```python
from build123d import *

# Parameters (mm, degrees)
RESSALTO_EXTRUS_O1_DEPTH  = 5
RESSALTO_EXTRUS_O2_DEPTH  = 15.5
RESSALTO_EXTRUS_O3_DEPTH  = 15.5
RESSALTO_EXTRUS_O4_DEPTH  = 20
ESBO_O6_W                 = 5
ESBO_O6_H                 = 16.897720337
RESSALTO_EXTRUS_O5_DEPTH  = 23.2
ESBO_O7_W                 = 13.499987793
ESBO_O7_H                 = 16.897720337
RESSALTO_EXTRUS_O6_DEPTH  = 8
ESBO_O8_W                 = 2.000000014
ESBO_O8_H                 = 6.588073731
CORTE_EXTRUS_O1_DEPTH     = 93.188310305
CHANFRO2_SIZE             = 9
RESSALTO_EXTRUS_O8_DEPTH  = 4.5
RESSALTO_EXTRUS_O7_START  = -5.5
RESSALTO_EXTRUS_O7_DEPTH  = 6
CORTE_EXTRUS_O2_REACH     = 102.674
ESBO_O11_W                = 11.999984741
ESBO_O11_H                = 13.640792847
CORTE_EXTRUS_O4_REACH     = 108.65
ESBO_O13_R                = 1.6
RESSALTO_EXTRUS_O9_DEPTH  = 5
ESBO_O16_W                = 11.500915527
ESBO_O16_H                = 13.642723083
CORTE_EXTRUS_O5_DEPTH     = 101.673633611
RESSALTO_EXTRUS_O13_START = -15.5
ESBO_O18_W                = 32.102264404
ESBO_O18_H                = 11
RESSALTO_EXTRUS_O13_DEPTH = 77.5
ESBO_O27_W                = 32.102264404
ESBO_O27_H                = 11
CORTE_EXTRUS_O8_DEPTH     = 20.5
ESBO_O29_R                = 1.9
CORTE_EXTRUS_O9_DEPTH     = 2.5
ESBO_O30_R                = 1.9
CORTE_EXTRUS_O10_DEPTH    = 6
ESBO_O32_W                = 20
ESBO_O32_H                = 78
CORTE_EXTRUS_O11_DEPTH    = 88.462468019
ESBO_O33_R                = 1.75
CORTE_EXTRUS_O12_DEPTH    = 26
CORTE_EXTRUS_O13_START    = -6
CORTE_EXTRUS_O13_DEPTH    = 2.9
RESSALTO_EXTRUS_O20_DEPTH = 10
ESBO_O40_W                = 68.75
ESBO_O40_H                = 49.5
ESBO_O40_W_2              = 60.75
ESBO_O40_H_2              = 41.5
RESSALTO_EXTRUS_O21_DEPTH = 18.5
ESBO_O41_W                = 11.75
ESBO_O41_H                = 49.5
ESBO_O41_W_2              = 41.5
ESBO_O41_H_2              = 38.5
RESSALTO_EXTRUS_O22_DEPTH = 2
RESSALTO_EXTRUS_O23_DEPTH = 15.5
ESBO_O43_W                = 4
ESBO_O43_H                = 33.5
ESBO_O43_W_2              = 14
ESBO_O43_H_2              = 4
CORTE_EXTRUS_O14_DEPTH    = 18.5
RESSALTO_EXTRUS_O24_DEPTH = 20.5
ESBO_O45_R                = 1.8
CORTE_EXTRUS_O15_DEPTH    = 6
FILETE1_R                 = 4
FILETE2_R                 = 2


with BuildPart() as part:
    # Esboço2 → Ressalto-extrusão1 (new body)
    with BuildSketch(Plane.XY):
        Polygon((0, 0), (0, -60.9), (-20, -60.9), (-20, -25.9), (-15.5, -15.9), (-15.5, 0), align=None)
    extrude(amount=RESSALTO_EXTRUS_O1_DEPTH)

    # Esboço3 → Ressalto-extrusão2 (add)
    with BuildSketch(Plane(origin=(0, 0, 0), x_dir=(0, 0, -1), z_dir=(1, 0, 0))):
        with BuildLine():
            ThreePointArc((6.102294922, 14.1), (-2.871049482, 9.744626932), (-5, 0))
            Line((-5, 0), (0, 0))
            ThreePointArc((0, 0), (1.788130128, 4.313492501), (6.102294922, 6.1))
            Line((6.102294922, 6.1), (30.102294922, 6.1))
            ThreePointArc((30.102294922, 6.099999986), (40.781022689, 1.676452573), (45.204559313, -9.002279663))
            Line((45.204559326, -9.002279663), (45.204559326, -60.9))
            Line((45.204559326, -60.9), (50.204559326, -60.9))
            Line((50.204559326, -60.9), (50.204559326, 14.1))
            Line((50.204559326, 14.1), (6.102294922, 14.1))
        make_face()
    extrude(amount=-RESSALTO_EXTRUS_O2_DEPTH)

    # Esboço4 → Ressalto-extrusão3 (add)
    with BuildSketch(Plane.ZY.offset(15.5)):
        Polygon((-50.204559326, -60.9), (-50.204559326, -40.9), (-65.204559326, -50.9), (-65.204559326, -60.9), align=None)
    extrude(amount=-RESSALTO_EXTRUS_O3_DEPTH)

    # Esboço5 → Ressalto-extrusão4 (add)
    with BuildSketch(Plane.ZY.offset(20)):
        Polygon((5, -60.9), (20, -60.9), (20, -50.9), (5, -40.9), align=None)
    extrude(amount=-RESSALTO_EXTRUS_O4_DEPTH)

    # Esboço6 → Ressalto-extrusão5 (add)
    with BuildSketch(Plane.ZY.offset(15.5)):
        with Locations((-47.704559326, -52.451139832)):
            Rectangle(ESBO_O6_W, ESBO_O6_H)
    extrude(amount=RESSALTO_EXTRUS_O5_DEPTH)

    # Esboço7 → Ressalto-extrusão6 (add)
    with BuildSketch(Plane.XY.offset(-45.204559326)):
        with Locations((-31.950006104, -52.451139832)):
            Rectangle(ESBO_O7_W, ESBO_O7_H)
    extrude(amount=RESSALTO_EXTRUS_O6_DEPTH)

    # Esboço8 → Corte-extrusão1 (cut, through all)
    with BuildSketch(Plane.ZY.offset(15.5)):
        with Locations((-46.204559319, -12.296316529)):
            Rectangle(ESBO_O8_W, ESBO_O8_H)
    extrude(amount=-CORTE_EXTRUS_O1_DEPTH, mode=Mode.SUBTRACT)

    # Chanfro2
    # the kernel refuses this chamfer: 9 mm, written as the material it adds along each edge
    with BuildSketch(Plane(origin=(-15.5, -44.002279663, -50.204559326), x_dir=(0.027495876610586407, 0.9996219169112969, 0), z_dir=(0, 0, 1))) as chanfro2_piece_1:
        Polygon((CHANFRO2_SIZE * 0.999621916911, CHANFRO2_SIZE * 0.0274958766106), (-CHANFRO2_SIZE * 0.0274958766106, CHANFRO2_SIZE * 0.999621916911), (0, 0), align=None)
    extrude(amount=5)

    # Esboço10 → Ressalto-extrusão8 (add)
    with BuildSketch(Plane.ZY.offset(15.5)):
        Polygon((-50.204559326, -40.9), (-50.204559326, -60.9), (-65.204559326, -60.9), (-65.204559326, -50.9), align=None)
    extrude(amount=RESSALTO_EXTRUS_O8_DEPTH)

    # Esboço9 → Ressalto-extrusão7 (add)
    with BuildSketch(Plane.XZ.offset(60.9).offset(RESSALTO_EXTRUS_O7_START)):
        Polygon((-38.7, -50.204559326), (-38.700004578, -53.204559326), (-20, -59.204559326), (-20, -50.204559326), align=None)
    extrude(amount=-RESSALTO_EXTRUS_O7_DEPTH)

    # Corte-extrusão2: up to this face of the body (flat: up to its plane)
    corte_extrus_o2_end = Plane(part.part.faces().sort_by_distance((-10, -45.9, 12.5))[0])
    # Esboço11 → Corte-extrusão2 (cut, up to the picked face)
    with BuildSketch(Plane.XY.offset(5), mode=Mode.PRIVATE) as corte_extrus_o2_sk1:
        with Locations((-10.00000763, -47.720396424)):
            Rectangle(ESBO_O11_W, ESBO_O11_H)
    corte_extrus_o2_tool1 = split(extrude(corte_extrus_o2_sk1.sketch, amount=CORTE_EXTRUS_O2_REACH, mode=Mode.PRIVATE), bisect_by=corte_extrus_o2_end, keep=Keep.BOTH, mode=Mode.PRIVATE)
    add(corte_extrus_o2_tool1.solids().sort_by(Axis((-10.000008, -47.720396, 5), (0, 0, 1)))[0], mode=Mode.SUBTRACT)

    # Esboço13 → Corte-extrusão4 (cut, up to next)
    with BuildSketch(Plane.XZ.offset(60.9), mode=Mode.PRIVATE) as corte_extrus_o4_sk1:
        with Locations(Location((-10, 12.5, 0), (0, 0, 270))):
            Circle(ESBO_O13_R)
    corte_extrus_o4_tool1 = extrude(corte_extrus_o4_sk1.sketch, amount=-CORTE_EXTRUS_O4_REACH, mode=Mode.PRIVATE) & part.part
    # Esboço13 → Corte-extrusão4 (cut, up to next)
    with BuildSketch(Plane.XZ.offset(60.9), mode=Mode.PRIVATE) as corte_extrus_o4_sk2:
        with Locations(Location((-9.7, -57.704559326, 0), (0, 0, 270))):
            Circle(ESBO_O13_R)
    corte_extrus_o4_tool2 = extrude(corte_extrus_o4_sk2.sketch, amount=-CORTE_EXTRUS_O4_REACH, mode=Mode.PRIVATE) & part.part
    add(corte_extrus_o4_tool1.solids().sort_by_distance((-10, -60.9, 12.5))[0], mode=Mode.SUBTRACT)
    add(corte_extrus_o4_tool2.solids().sort_by_distance((-9.7, -60.9, -57.704559))[0], mode=Mode.SUBTRACT)

    # Esboço14 → Ressalto-extrusão9 (add)
    with BuildSketch(Plane.XY.offset(5)):
        Polygon((-10.75, 0), (-4.75, 0), (-4.75, -15.9), (-7.000007629, -25.9), (-7.000007629, -40.9), (-13.000007629, -40.9), (-13.000007629, -25.9), (-10.75, -15.9), align=None)
    extrude(amount=RESSALTO_EXTRUS_O9_DEPTH)

    # Esboço16 → Corte-extrusão5 (cut, through all)
    with BuildSketch(Plane(origin=(0, 0, -50.204559326), x_dir=(-1, 0, 0), z_dir=(0, 0, -1))):
        with Locations((9.750457764, -47.721361542)):
            Rectangle(ESBO_O16_W, ESBO_O16_H)
    extrude(amount=CORTE_EXTRUS_O5_DEPTH, mode=Mode.SUBTRACT)

    # Esboço18 → Ressalto-extrusão13 (add)
    with BuildSketch(Plane(origin=(0, 0, 0), x_dir=(0, 0, -1), z_dir=(1, 0, 0)).offset(RESSALTO_EXTRUS_O13_START)):
        with Locations((34.153427124, 11.6)):
            Rectangle(ESBO_O18_W, ESBO_O18_H)
    extrude(amount=RESSALTO_EXTRUS_O13_DEPTH)

    # Esboço27 → Corte-extrusão8 (cut)
    with BuildSketch(Plane(origin=(62, 0, 0), x_dir=(0, 0, -1), z_dir=(1, 0, 0))):
        with Locations((34.153427124, 11.6)):
            Rectangle(ESBO_O27_W, ESBO_O27_H)
    extrude(amount=-CORTE_EXTRUS_O8_DEPTH, mode=Mode.SUBTRACT)

    # Esboço29 → Corte-extrusão9 (cut)
    with BuildSketch(Plane(origin=(41.5, 0, 0), x_dir=(0, 0, -1), z_dir=(1, 0, 0))):
        with Locations((22.364620491, 9.524231873)):
            Circle(ESBO_O29_R)
        Polygon((24.102294922, 17.1), (22.486408956, 13.10054189), (18.102294922, 13.10054189), (18.102294922, 17.1), align=None)
    extrude(amount=-CORTE_EXTRUS_O9_DEPTH, mode=Mode.SUBTRACT)

    # Esboço30 → Corte-extrusão10 (cut)
    with BuildSketch(Plane(origin=(0, 17.1, 0), x_dir=(1, 0, 0), z_dir=(0, 1, 0))):
        with Locations(Location((-10.5, 22.602294922, 0), (0, 0, 180))):
            Circle(ESBO_O30_R)
        with Locations(Location((24.5, 22.602294922, 0), (0, 0, 180))):
            Circle(ESBO_O30_R)
    extrude(amount=-CORTE_EXTRUS_O10_DEPTH, mode=Mode.SUBTRACT)

    # Esboço32 → Corte-extrusão11 (cut, through all)
    with BuildSketch(Plane.XY.offset(-18.102294922)):
        with Locations((-10, -21.9)):
            Rectangle(ESBO_O32_W, ESBO_O32_H)
    extrude(amount=CORTE_EXTRUS_O11_DEPTH, mode=Mode.SUBTRACT)

    # Esboço33 → Corte-extrusão12 (cut)
    with BuildSketch(Plane.XY.offset(-18.102294922)):
        with Locations((9, 11.6)):
            Circle(ESBO_O33_R)
        with Locations((33, 11.6)):
            Circle(ESBO_O33_R)
    extrude(amount=-CORTE_EXTRUS_O12_DEPTH, mode=Mode.SUBTRACT)

    # Esboço34 → Corte-extrusão13 (cut)
    with BuildSketch(Plane.XY.offset(-18.102294922).offset(CORTE_EXTRUS_O13_START)):
        Polygon((9, 15.179571669), (5.9, 13.389785834), (5.9, 9.810214166), (5.9, 6.1), (12.1, 6.1), (12.1, 9.810214166), (12.1, 13.389785834), align=None)
        Polygon((29.9, 6.1), (29.9, 9.810214166), (29.9, 13.389785834), (33, 15.179571669), (36.1, 13.389785834), (36.1, 9.810214166), (36.1, 6.1), align=None)
    extrude(amount=-CORTE_EXTRUS_O13_DEPTH, mode=Mode.SUBTRACT)

    # Esboço39 → Ressalto-extrusão20 (add)
    with BuildSketch(Plane(origin=(0, 0, -50.204559326), x_dir=(-1, 0, 0), z_dir=(0, 0, -1))):
        Polygon((-41.5, 17.1), (-41.5, 6.1), (0, 6.1), (0, -32.4), (15.5, -32.4), (15.5, 17.1), align=None)
    extrude(amount=RESSALTO_EXTRUS_O20_DEPTH)

    # Esboço40 → Ressalto-extrusão21 (add)
    with BuildSketch(Plane(origin=(0, 0, -60.204559326), x_dir=(-1, 0, 0), z_dir=(0, 0, -1))):
        with Locations((-7.125, -7.65)):
            Rectangle(ESBO_O40_W, ESBO_O40_H)
        with Locations((-7.125, -7.65)):
            Rectangle(ESBO_O40_W_2, ESBO_O40_H_2, mode=Mode.SUBTRACT)
    extrude(amount=RESSALTO_EXTRUS_O21_DEPTH)

    # Esboço41 → Ressalto-extrusão22 (add)
    with BuildSketch(Plane.XY.offset(-60.204559326)):
        with Locations((-21.375, -7.65)):
            Rectangle(ESBO_O41_W, ESBO_O41_H)
        with Locations((20.75, -13.15)):
            Rectangle(ESBO_O41_W_2, ESBO_O41_H_2)
    extrude(amount=RESSALTO_EXTRUS_O22_DEPTH)

    # Esboço42 → Ressalto-extrusão23 (add)
    with BuildSketch(Plane(origin=(41.5, 0, 0), x_dir=(0, 0, -1), z_dir=(1, 0, 0))):
        with BuildLine():
            Line((45.204559312, -9.002279663), (58.204559326, -9.002279663))
            Line((58.204559326, -9.002279663), (58.204559326, 6.1))
            Line((58.204559326, 6.1), (30.101642126, 6.1))
            ThreePointArc((30.101642126, 6.1), (40.780791888, 1.676683369), (45.204559312, -9.002279663))
        make_face()
    extrude(amount=-RESSALTO_EXTRUS_O23_DEPTH)

    # Esboço43 → Corte-extrusão14 (cut)
    with BuildSketch(Plane(origin=(0, 0, -78.704559326), x_dir=(-1, 0, 0), z_dir=(0, 0, -1))):
        with Locations((-39.5, -7.65)):
            Rectangle(ESBO_O43_W, ESBO_O43_H)
        with Locations((25.25, -7.65)):
            Rectangle(ESBO_O43_W, ESBO_O43_H)
        with Locations((-22.5, 15.1)):
            Rectangle(ESBO_O43_W_2, ESBO_O43_H_2)
    extrude(amount=-CORTE_EXTRUS_O14_DEPTH, mode=Mode.SUBTRACT)

    # Esboço44 → Ressalto-extrusão24 (add)
    with BuildSketch(Plane(origin=(0, 0, -78.704559326), x_dir=(-1, 0, 0), z_dir=(0, 0, -1))):
        with BuildLine():
            Line((-43.5, 17.1), (-41.5, 17.1))
            Line((-41.5, 17.1), (-41.5, 9.1))
            Line((-41.5, 9.1), (-43.5, 9.1))
            ThreePointArc((-43.5, 9.1), (-47.5, 13.1), (-43.5, 17.1))
        make_face()
        with BuildLine():
            Line((29.25, -24.4), (27.25, -24.4))
            Line((27.25, -24.4), (27.25, -32.4))
            Line((27.25, -32.4), (29.25, -32.4))
            ThreePointArc((29.25, -32.4), (33.25, -28.4), (29.25, -24.4))
        make_face()
    extrude(amount=-RESSALTO_EXTRUS_O24_DEPTH)

    # Esboço45 → Corte-extrusão15 (cut)
    with BuildSketch(Plane(origin=(0, 0, -78.704559326), x_dir=(-1, 0, 0), z_dir=(0, 0, -1))):
        with Locations(Location((-43.5, 13.1, 0), (0, 0, 90))):
            Circle(ESBO_O45_R)
        with Locations(Location((29.25, -28.4, 0), (0, 0, 90))):
            Circle(ESBO_O45_R)
    extrude(amount=-CORTE_EXTRUS_O15_DEPTH, mode=Mode.SUBTRACT)

    # Filete1
    filete1_edges = [part.edges().sort_by_distance(p)[0] for p in [
        (-15.5, -7.65, -58.204559326),
    ]]
    fillet(filete1_edges, radius=FILETE1_R)

    # Filete2
    filete2_edges = [part.edges().sort_by_distance(p)[0] for p in [
        (-7.75, -32.4, -50.204559326),
    ]]
    fillet(filete2_edges, radius=FILETE2_R)


solid = part.part
```
Check sheet for the modelled part. Datum: model origin and axes. Units: mm. A direction names the side the tool comes from. Give positions to 0.01 mm unless a question says otherwise; leave off trailing zeros. Write each loop counter-clockwise with the first axis right and the second up, starting at its lowest first coordinate (ties: lowest second). Pieces come first, ordered by that corner, then holes.
Item 1: Scan lines: L1, parallel to Y at x = 9, z = -34.75; L2, parallel to X at y = 6, z = -38; L3, parallel to Y at x = -16, z = -64. Record each from-to range of solid material in increasing order.
Item 2: Cross-section at B-B (y = -42). Enter the section's corners in (x, z), and give its area (3 significant figures).
Item 3: Gauge pin test, flat ends, axial feed: pin 1 (1.2 mm diameter, centred on x = -25, z = -71, fed in from -Y); pin 2 (6 mm diameter, centred on x = -16, z = -38.5, fed in from -Y); pin 3 (2 mm diameter, centred on x = 37.5, z = -45, fed in from -Y); pin 4 (2 mm diameter, centred on y = -8.5, z = -63, fed in from +X). Record the tip position at first contact, or that the pin passes through.
Item 4: Cross-section at C-C (x = -6.5). Enter the section's corners in (y, z).
Item 5: Draft check along X on faces 1 (the face through (-33.25, -28.49, -68.6)), 2 (the face through (8, -28.4, -69)), 3 (the face through (-1.97, -45.97, -57.81)). Enter one of: released by +X, released by -X, zero draft, split by the parting line, or undercut.
Item 6: Cross-section at A-A (x = 18.5). Enter the section's corners in (y, z).
Item 7: Access from +Z, -Z, +X, -X, +Y, -Y to the whole of each face (thin tool, end or side, straight path). Record for faces 4 (the face through (-4, -49, -56)), 5 (the face through (-10, -39, -45.205)), 6 (the face through (9, 12, -44.102)), 7 (the face through (-10, -57, -65.205)), 8 (the face through (6, -32.4, -69)).
Report:
1. L1: y = 6.1 to 9.85, 13.35 to 17.1
1. L2: x = -15.5 to 0, 26 to 41.5
1. L3: y = -60.9 to -50.1, -32.4 to -28.4, 13.1 to 17.1
2. outline: (-22.5, -50.2) - (-20, -50.2) - (-20, -51.85) - (-15.5, -51.85) - (-15.5, -50.2) - (-4, -50.2) - (-4, -51.85) - (0, -51.85) - (0, -45.2) - (-22.5, -45.2) - close
2. area: 127 mm2
3. pin 1: stops at y = -32.4
3. pin 2: stops at y = 0.95
3. pin 3: stops at y = -9
3. pin 4: passes through
4. outline: (-60.9, -65.2) - (-54.54, -65.2) - (-54.54, -50.2) - (-34.4, -50.2) arc R2 cw to (-32.4, -52.2) - (-32.4, -78.7) - (-28.4, -78.7) - (-28.4, -60.2) - (13.1, -60.2) - (13.1, -78.7) - (17.1, -78.7) - (17.1, -18.1) - (6.1, -18.1) - (6.1, -30.1) arc R15.1 cw to (-9, -45.2) - (-9, -47.2) - (-15.59, -47.2) - (-15.59, -45.2) - (-60.9, -45.2) - close
5. face 1: released by -X
5. face 2: undercut
5. face 3: zero draft
6. outline: (-32.4, -78.7) - (-28.4, -78.7) - (-28.4, -60.2) - (17.1, -60.2) - (17.1, -18.1) - (6.1, -18.1) - (6.1, -58.2) - (-32.4, -58.2) - close
7. face 4: -Z
7. face 5: +Z, +X, -Y
7. face 6: +Z
7. face 7: -Z, +X, -X, -Y
7. face 8: -Z, +X, -X
